CAD build for the part. Positions are in the model's coordinates, mm. Give positions to 0.01 mm unless a question says otherwise; leave off trailing zeros. Loops run counter-clockwise (first coordinate to the right, second up) from the corner with the lowest first, then second, coordinate; pieces in that order, holes last. Notation, with made-up numbers: (68, 88) - (91, 88) arc R15 ccw to (91, 109) - close; hole circle Ø5 at (-39.5, -38.5). An arc over 180 degrees is marked (long way). Return JSON: item names as keys, results as strings.
Autodesk Inventor part; units mm, degrees
ref_plane "YZ Plane" through (0, 0, 0) normal (1, 0, 0) x (0, 1, 0)
ref_plane "XZ Plane" through (0, 0, 0) normal (0, 1, 0) x (-1, 0, 0)
ref_plane "XY Plane" through (0, 0, 0) normal (0, 0, 1) x (1, 0, 0)
sketch "Sketch1" plane through (0, 0, 0) normal (1, 0, 0) x (0, 1, 0)
  line L0 (15, 0) -> (165, 0)
  line L1 (180, 15) -> (180, 165)
  line L2 (165, 180) -> (15, 180)
  line L3 (0, 165) -> (0, 15)
  line L4 (180, 180) -> (0, 0) construction
  line L5 (30, 30) -> (150, 30) construction
  line L6 (150, 30) -> (150, 150) construction
  line L7 (150, 150) -> (30, 150) construction
  line L8 (30, 150) -> (30, 30) construction
  line L9 (30, 30) -> (150, 150) construction
  line L10 (150, 30) -> (30, 150) construction
  line L11 (37.5, 37.5) -> (142.5, 37.5) construction
  line L12 (142.5, 37.5) -> (142.5, 142.5) construction
  line L13 (142.5, 142.5) -> (37.5, 142.5) construction
  line L14 (37.5, 142.5) -> (37.5, 37.5) construction
  line L15 (37.5, 37.5) -> (142.5, 142.5) construction
  line L16 (142.5, 37.5) -> (37.5, 142.5) construction
  circle A0 centre (142.5, 142.5) radius 2
  circle A1 centre (142.5, 37.5) radius 2
  circle A2 centre (37.5, 37.5) radius 2
  circle A3 centre (37.5, 142.5) radius 2
  circle A4 centre (90, 90) radius 62.5
  arc A5 (180, 165) -> (165, 180) centre (165, 165) ccw
  arc A6 (165, 0) -> (180, 15) centre (165, 15) ccw
  arc A7 (0, 15) -> (15, 0) centre (15, 15) ccw
  arc A8 (15, 180) -> (0, 165) centre (15, 165) ccw
  line L17 (7.5, 7.5) -> (172.5, 7.5) construction
  line L18 (172.5, 7.5) -> (172.5, 172.5) construction
  line L19 (172.5, 172.5) -> (7.5, 172.5) construction
  line L20 (7.5, 172.5) -> (7.5, 7.5) construction
  line L21 (7.5, 7.5) -> (172.5, 172.5) construction
  line L22 (172.5, 7.5) -> (7.5, 172.5) construction
  circle A9 centre (172.5, 172.5) radius 2
  circle A10 centre (172.5, 7.5) radius 2
  circle A11 centre (7.5, 7.5) radius 2
  circle A12 centre (7.5, 172.5) radius 2
  dimension "d0" = 180
  dimension "d1" = 180
  dimension "d2" = 120
  dimension "d3" = 105
  dimension "d4" = 4
  dimension "d5" = 125
  dimension "d6" = 15
  dimension "d9" = 4
  dimension "d10" = 165
extrude "Extrusion1" add sketch "Sketch1" along normal blind 2.75
sketch "Sketch2" plane through (2.75, 0, 0) normal (1, 0, 0) x (0, 0, -1)
  circle A0 centre (-22.5, 164.5) radius 7.5
  circle A1 centre (-7.5, 172.5) radius 2
  point P0 (0, 0)
  dimension "d11" = 15
  dimension "d12" = 15
  dimension "d13" = 8
extrude "Extrusion2" cut sketch "Sketch2" against normal blind 10 contours A0
properties part number "TrayPanelD_120mmAdapter"
1. Pull direction Z, two halves, no side cores. Call faces 1 (the face through (1.36, 4.28, 175.49)), 2 (the face through (0, 69, 151)), 3 (the face through (1.356, 5.502, 7.412)), 4 (the face through (1.356, 8.423, 174.274)): +Z half, -Z half, draft (parallel to the pull), parting line (faces both ways), or undercut.
Values follow:
{"face 1": "+Z half", "face 2": "draft", "face 3": "undercut", "face 4": "undercut"}
2. Drill centre lines: probe 1 along Y at (x, z) = (2.05, 22.5); probe 2 along Y at (x, z) = (1.45, 142.5). Where is each one in solid material? Low to high.
Values follow:
{"probe 1": "y = 0 to 157, 172 to 180", "probe 2": "y = 0 to 35.5, 39.5 to 56.09, 123.91 to 140.5, 144.5 to 180"}
3. Cut at A-A, the plane y = 90. Write the cut outline in (x, z).
Values follow:
{"outline": "(0, 0) - (2.75, 0) - (2.75, 27.5) - (0, 27.5) - close; (0, 152.5) - (2.75, 152.5) - (2.75, 180) - (0, 180) - close"}
4. Drop flat-ended pins along their axis: P1, Ø1.5, axis at x = 2, y = 26.5, coming from the -Z side; P2, Ø2.5, axis at y = 172.5, z = 172.5, coming from the -X side. Give the stop position or say it passes through.
Values follow:
{"P1": "stops at z = 0", "P2": "passes through"}
5. Cut at C-C, the plane z = 111. Write the cut outline in (x, y).
Values follow:
{"outline": "(0, 0) - (2.75, 0) - (2.75, 31.13) - (0, 31.13) - close; (0, 148.87) - (2.75, 148.87) - (2.75, 180) - (0, 180) - close"}
6. Cut at B-B, the plane x = 1.95. Give the number of separate pieces and of enclosed holes in the cut face, plus the area to 3 significant figures.
Values follow:
{"separate pieces": "1", "enclosed holes": "10", "area": "19,700 mm²"}
